```python
from build123d import *

# Parameters (mm, degrees)
F0_W     = 80
F0_H     = 50
F1_DEPTH = 80
F2_SIZE  = 5
F3_T     = -2.5


with BuildPart() as f1:
    # F0 (on Top) → F1 (new body)
    with BuildSketch(Plane.XY):
        with Locations((-8.405441, -0.035937)):
            Rectangle(F0_W, F0_H)
    extrude(amount=F1_DEPTH)

    # F2
    f2_edges = [f1.edges().sort_by_distance(p)[0] for p in [
        (31.594559, -0.035937, 80),
        (31.594559, -25.035937, 40),
        (31.594559, -0.035937, 0),
        (31.594559, 24.964063, 40),
        (-48.405441, -0.035937, 80),
        (-48.405441, 24.964063, 40),
        (-8.405441, 24.964063, 0),
        (-8.405441, 24.964063, 80),
        (-8.405441, -25.035937, 80),
        (-48.405441, -0.035937, 0),
        (-8.405441, -25.035937, 0),
        (-48.405441, -25.035937, 40),
    ]]
    chamfer(f2_edges, length=F2_SIZE)

    # F3
    f3_openings = [f1.faces().sort_by_distance(p)[0] for p in [
        (-8.405441, 24.964063, 40),
    ]]
    offset(amount=F3_T, openings=f3_openings)


solid = f1.part
```
Can you work these out from the model? Positions are in its coordinate system, mm. A direction names the side the tool comes from. Coordinates: 2 decimals unless noted, no trailing zeros. Loops run counter-clockwise (first coordinate to the right, second up) from the corner with the lowest first, then second, coordinate; pieces in that order, holes last. Notation, with made-up numbers: (-2, 48.25) - (38, 48.25) arc R27 ccw to (38, 78.25) - close; hole circle Ø3 at (4.25, 59). An arc over 180 degrees is marked (long way). Answer as CSV lines item,"result". Start each with the question number.
1) Suppose I cut it at A-A (z = 52). Please give me the cut outline in (x, y).
2) Suppose I cut it at C-C (x = -33). Please give me the cut outline in (y, z).
3) Suppose I cut it at B-B (y = -13.5). Please give me the cut outline in (x, z).
4) For pin 1 (5 mm diameter, centred on x = 5, z = 54, fed in from +Y), with a flat end and sliding along its axis, tell me the tip position at first contact or that it passes through.
5) Thinking about a two-plate mould opening in Y: for faces 1 (the flat face through (-8.895, -22.501, 2.465)), 2 (the flat face through (-45.87, -0.316, 2.465)), 3 (the flat face through (-43.53, -20.41, 75.17)), which applies, pulls with the +Y half, pulls with the -Y half, needs draft (parallel to the pull), parting line crosses it, or undercut?
6) I need wall thicknesses on line 1 (Z direction, x = -21, y = 16); line 2 (X direction, y = -6, z = 59); line 3 (Y direction, x = -25.5, z = 11.5). Which ranges of each line are inside material? Lowest first, please. Write a range as from..to.
7) Which directions (+Z, -Z, +X, -X, +Y, -Y) give clear straight access to the entire face, cutting with the end or side of a thin tool? Please do faces 4 (the flat face through (-8.895, 22.429, 77.535)), 5 (the flat face through (26.765, 20.336, 4.872)).
Check result:
1,outline,"(-48.41, -20.04) - (-43.41, -25.04) - (26.59, -25.04) - (31.59, -20.04) - (31.59, 19.96) - (26.59, 24.96) - (23.06, 24.96) - (29.09, 18.93) - (29.09, -19) - (25.56, -22.54) - (-42.37, -22.54) - (-45.91, -19) - (-45.91, 18.93) - (-39.87, 24.96) - (-43.41, 24.96) - (-48.41, 19.96) - close"
2,outline,"(-25.04, 5) - (-20.04, 0) - (19.96, 0) - (24.96, 5) - (24.96, 8.54) - (18.93, 2.5) - (-19, 2.5) - (-22.54, 6.04) - (-22.54, 73.96) - (-19, 77.5) - (18.93, 77.5) - (24.96, 71.46) - (24.96, 75) - (19.96, 80) - (-20.04, 80) - (-25.04, 75) - close"
3,outline,"(-48.41, 5) - (-43.41, 0) - (26.59, 0) - (31.59, 5) - (31.59, 75) - (26.59, 80) - (-43.41, 80) - (-48.41, 75) - close; hole (-45.91, 6.04) - (-42.37, 2.5) - (25.56, 2.5) - (29.09, 6.04) - (29.09, 73.96) - (25.56, 77.5) - (-42.37, 77.5) - (-45.91, 73.96) - close"
4,pin 1,"stops at y = -22.54"
5,face 1,"pulls with the -Y half"
5,face 2,"needs draft"
5,face 3,"undercut"
6,line 1,"z = 0..2.5, 77.5..80"
6,line 2,"x = -48.41..-45.91, 29.09..31.59"
6,line 3,"y = -25.04..-22.54"
7,face 4,"+Z, +X, -X, +Y"
7,face 5,"none"
